Input: part model. Units: mm. Frame: model coordinates. Face numbers are marked on the shaded views. Round coordinates to 2 decimals unless told otherwise and drop trailing zeros. Write each loop counter-clockwise with the first axis right and the second up, starting at its lowest first coordinate (ties: lowest second). Pieces come first, ordered by that corner, then holes. Notation, with made-up numbers: M 61,-6 L 74,-6 A29 cw 74,18 Z; hole C -37,76.5 d8. An arc over 180 degrees is marked long. Use one line per item in the form item = value. Start each with the question number.
```python
from build123d import *

# Parameters (mm, degrees)
SKETCH1_W           = 70
SKETCH1_H           = 65
SKETCH1_W_2         = 66
SKETCH1_H_2         = 61
BOSS_EXTRUDE1_DEPTH = 5
SKETCH2_W           = 66
SKETCH2_H           = 61
BOSS_EXTRUDE2_DEPTH = 2
FILLET2_R           = 2


with BuildPart() as part:
    # Sketch1 → Boss-Extrude1 (new body)
    with BuildSketch(Plane(origin=(0, 0, 0), x_dir=(1, 0, 0), z_dir=(0, 1, 0))):
        Rectangle(SKETCH1_W, SKETCH1_H)
        Rectangle(SKETCH1_W_2, SKETCH1_H_2, mode=Mode.SUBTRACT)
    extrude(amount=BOSS_EXTRUDE1_DEPTH)

    # Sketch2 → Boss-Extrude2 (add)
    with BuildSketch(Plane(origin=(0, 0, 0), x_dir=(1, 0, 0), z_dir=(0, 1, 0))):
        Rectangle(SKETCH2_W, SKETCH2_H)
    extrude(amount=BOSS_EXTRUDE2_DEPTH)

    # Fillet2
    fillet2_edges = [part.edges().sort_by_distance(p)[0] for p in [
        (0, 0, 32.5),
        (-35, 0, 0),
        (0, 0, -32.5),
        (35, 0, 0),
        (35, 2.5, 32.5),
        (-35, 2.5, 32.5),
        (-35, 2.5, -32.5),
        (35, 2.5, -32.5),
    ]]
    fillet(fillet2_edges, radius=FILLET2_R)


solid = part.part
```
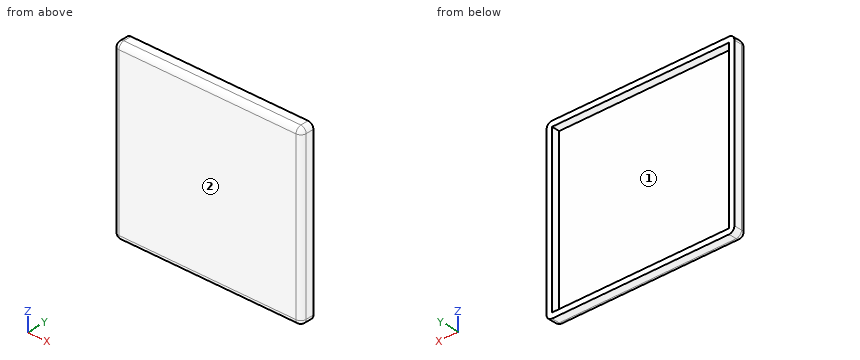
Item 1: Cut plane A-A (y = 4.25). Output: boundary loops of the cut face in (x, z).
Item 2: Draft query along X for the marked faces 1 and 2. Return one class per face: +X half, -X half, draft (parallel to the pull), parting line (faces both ways), or undercut.
Item 3: First-contact query: pin 1 (4 mm diameter, centred on x = -1, z = 24.5, fed in from +Y). Flat tip, straight axial feed; report the tip coordinate or a pass-through.
Item 4: Cut plane C-C (z = -2). Output: boundary loops of the cut face in (x, y).
Item 5: Ray query, line 1 (Z direction, x = 18.5, y = 2.15); line 2 (X direction, y = 3.7, z = 14.5); line 3 (Y direction, x = 17.5, z = 10). Return the intervals inside material, ascending. Write a range as from..to.
Item 6: Cut plane B-B (x = -30.5). Output: boundary loops of the cut face in (y, z).
Final values:
q1.outline = M -35,-30.5 A2 ccw -33,-32.5 L 33,-32.5 A2 ccw 35,-30.5 L 35,30.5 A2 ccw 33,32.5 L -33,32.5 A2 ccw -35,30.5 Z; hole M -33,-30.5 L 33,-30.5 L 33,30.5 L -33,30.5 Z
q2.face_1 = undercut
q2.face_2 = draft
q3.pin_1 = 2
q4.outline = M -35,2 A2 ccw -33,0 L 33,0 A2 ccw 35,2 L 35,5 L 33,5 L 33,2 L -33,2 L -33,5 L -35,5 Z
q5.line_1 = -32.5..-30.5, 30.5..32.5
q5.line_2 = -35..-33, 33..35
q5.line_3 = 0..2
q6.outline = M 0,-30.5 A2 ccw 2,-32.5 L 5,-32.5 L 5,-30.5 L 2,-30.5 L 2,30.5 L 5,30.5 L 5,32.5 L 2,32.5 A2 ccw 0,30.5 Z
